Geometry check sheet. Reference: the model listing, model coordinates, mm. Give positions to 0.01 mm unless a question says otherwise; leave off trailing zeros. Order: outer loops, then holes, each group sorted by start corner. A loop starts at its lowest first (then second) coordinate and runs counter-clockwise, first axis right, second up. Notation, with made-up numbers: M 81.25,74.5 L 112.25,74.5 A23 ccw 112.25,102.5 Z; hole C 17.5,32 d1. An arc over 180 degrees is marked long. Answer as CSV lines item,"result". Start each with the question number.
Autodesk Fusion 360 part; units mm, degrees
sketch "ControlPanel" plane through (0, 0, 0) normal (0, 1, 0) x (-1, 0, 0)
  line L0 (0, 0) -> (73, 0)
  line L1 (73, 0) -> (73, 41)
  line L2 (73, 41) -> (0, 41)
  line L3 (0, 41) -> (0, 0)
  line L4 (-11.9813, -5) -> (34.0187, -5)
  line L5 (34.0187, -5) -> (34.0187, -32)
  line L6 (34.0187, -32) -> (-11.9813, -32)
  line L7 (-11.9813, -32) -> (-11.9813, -5)
  line L8 (77.6844, -83.0568) -> (77.6844, -82.5327)
  line L9 (-12.1589, -88.0054) -> (-12.1589, -100.8506)
  line L10 (13.8411, -100.8506) -> (13.8411, -88.0054)
  arc A0 (-12.1589, -100.8506) -> (13.8411, -100.8506) centre (0.8411, -94.428) ccw
  arc A1 (13.8411, -88.0054) -> (-12.1589, -88.0054) centre (0.8411, -94.428) ccw
  line L11 (76.8382, -83.928) -> (70.2808, -83.928)
  line L12 (63.0595, -91.1493) -> (63.0595, -97.7068)
  line L13 (70.2808, -104.928) -> (76.8382, -104.928)
  line L14 (84.0595, -97.7068) -> (84.0595, -91.1493)
  arc A2 (70.2808, -83.928) -> (63.0595, -91.1493) centre (73.5595, -94.428) ccw
  arc A3 (84.0595, -91.1493) -> (76.8382, -83.928) centre (73.5595, -94.428) ccw
  arc A4 (63.0595, -97.7068) -> (70.2808, -104.928) centre (73.5595, -94.428) ccw
  arc A5 (76.8382, -104.928) -> (84.0595, -97.7068) centre (73.5595, -94.428) ccw
  line L15 (39.0187, -5) -> (85.0187, -5)
  line L16 (85.0187, -5) -> (85.0187, -32)
  line L17 (85.0187, -32) -> (39.0187, -32)
  line L18 (39.0187, -32) -> (39.0187, -5)
  line L19 (-11.9813, -37) -> (34.0187, -37)
  line L20 (34.0187, -37) -> (34.0187, -64)
  line L21 (34.0187, -64) -> (-11.9813, -64)
  line L22 (-11.9813, -64) -> (-11.9813, -37)
  line L23 (39.0187, -37) -> (85.0187, -37)
  line L24 (85.0187, -37) -> (85.0187, -64)
  line L25 (85.0187, -64) -> (39.0187, -64)
  line L26 (39.0187, -64) -> (39.0187, -37)
  line L27 (34.0187, -5) -> (39.0187, -5) construction
  circle A6 centre (36.5, -94.428) radius 0.6723 construction
  line L28 (119.0595, -139.428) -> (119.0595, 71) construction
  line L29 (119.0595, 71) -> (-44.1589, 71) construction
  line L30 (-44.1589, 71) -> (-44.1589, -139.428) construction
  line L31 (-44.1589, 71) -> (119.0595, 71)
  line L32 (119.0595, 71) -> (119.0595, -219)
  line L33 (119.0595, -219) -> (-44.1589, -219)
  line L34 (-44.1589, -219) -> (-44.1589, 71)
  circle A7 centre (-14.1589, 61) radius 3
  circle A8 centre (89.0595, 61) radius 3
  circle A9 centre (-34.1589, 31) radius 3
  circle A10 centre (109.0551, 31) radius 3
  circle A11 centre (-34.1589, -19) radius 3
  circle A12 centre (109.0551, -19) radius 3
  circle A13 centre (-34.1589, -69) radius 3
  circle A14 centre (109.0551, -69) radius 3
  circle A15 centre (-34.1589, -119) radius 3
  circle A16 centre (109.0551, -119) radius 3
  circle A17 centre (-34.1589, -169) radius 3
  circle A18 centre (109.0551, -169) radius 3
  circle A19 centre (-14.1589, -209) radius 3
  circle A20 centre (89.0595, -209) radius 3
  point P0 (73.5595, -94.428)
  point P1 (0.8411, -94.428)
  point P2 (73.5595, -94.428)
  point P3 (0.8411, -94.428)
  point P4 (73.5595, -94.428)
  point P5 (-14.1589, -209)
  point P6 (89.0595, -209)
  dimension "d12" = 73
  dimension "d13" = 41
  dimension "d15" = 46
  dimension "d16" = 27
  dimension "d17" = 5
  dimension "d33" = 29
  dimension "d36" = 22
  dimension "d88" = 46
  dimension "d89" = 27
  dimension "d90" = 5
  dimension "d91" = 46
  dimension "d92" = 27
  dimension "d93" = 5
  dimension "d94" = 46
  dimension "d95" = 27
  dimension "d96" = 5
  dimension "d110" = 210.428
  dimension "d111" = 290
  dimension "d113" = 6
  dimension "d114" = 30
  dimension "d115" = 6
  dimension "d116" = 30
  dimension "d123" = 6
  dimension "d124" = 40
  dimension "d127" = 143.214
  dimension "d128" = -200
extrude "Extrude3" add sketch "ControlPanel" along normal blind 3 contours L31 L32 L33 L34 | A19 | A20
extrude "Extrude5" cut sketch "ControlPanel" along normal mid plane 12 contours A19
extrude "Extrude6" cut sketch "ControlPanel" along normal mid plane 12 contours A20
extrude "Extrude1" [suppressed]
equation "m2_w = 73 mm"
equation "m2_h = 41 mm"
equation "m1_w = 46 mm"
equation "m1_h = 27 mm"
equation "mpwr_dia = 12.2 mm"
equation "mpwr_key = 1 mm"
equation "reset_dia = 12.5 mm"
equation "apwr_dia = 29 mm"
equation "apwr_key = 26 mm"
equation "estop_dia = 22 mm"
equation "estop_key = 21 mm"
equation "d12 = m2_w"
equation "d13 = m2_h"
equation "meter_v = 5 mm"
equation "d15 = m1_w"
equation "d16 = m1_h"
equation "d17 = meter_v"
equation "apwr_shell = 37 mm"
equation "botrow_offset = 35 mm"
equation "d33 = apwr_dia"
equation "d36 = estop_dia"
equation "sw_dist = 100 mm"
equation "sw_offs = 25 mm"
equation "text_top_offs = 5 mm"
equation "d88 = m1_w"
equation "d89 = m1_h"
equation "d90 = meter_v"
equation "d91 = m1_w"
equation "d92 = m1_h"
equation "d93 = meter_v"
equation "d94 = m1_w"
equation "d95 = m1_h"
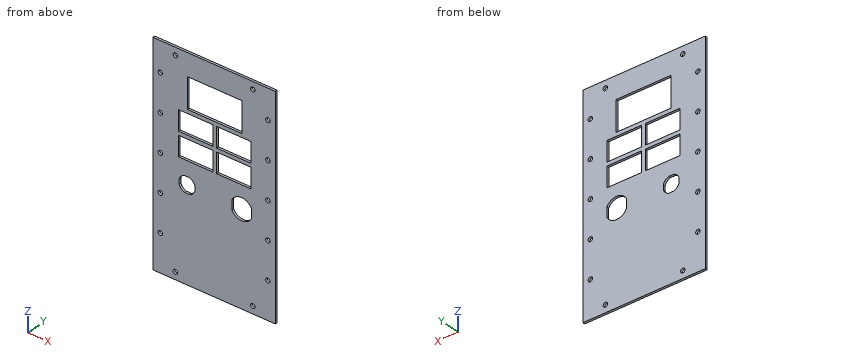
Item 1: Section check A-A on z = 31. Record the boundary of the cut face in (x, y), then the cut area to 3 significant figures.
Item 2: Section check C-C on z = -19. Record the boundary of the cut face in (x, y), then the cut area to 3 significant figures.
Item 3: Section check D-D on z = -169. Record the boundary of the cut face in (x, y), then the cut area to 3 significant figures.
Item 4: Section check B-B on x = -22. Record the boundary of the cut face in (y, z), then the cut area to 3 significant figures.
Item 5: Scan lines: line 1 along Z through (x, y) = (-27, 1.15); line 2 along Z through (x, y) = (34.5, 2); line 3 along X through (y, z) = (1.6, -57.5). Record each from-to range of solid material in increasing order.
Item 6: Depth check by flat-ended pin: pin 1 Ø3.5 at (x, z) = (-109.06, -19) entering from -Y. Enter the tip coordinate at first touch or a pass-through.
Numbers:
1,outline,"M -119.06,0 L -112.06,0 L -112.06,3 L -119.06,3 Z; M -106.06,0 L -73,0 L -73,3 L -106.06,3 Z; M 0,0 L 31.16,0 L 31.16,3 L 0,3 Z; M 37.16,0 L 44.16,0 L 44.16,3 L 37.16,3 Z"
1,area,"235 mm2"
2,outline,"M -119.06,0 L -112.06,0 L -112.06,3 L -119.06,3 Z; M -106.06,0 L -85.02,0 L -85.02,3 L -106.06,3 Z; M -39.02,0 L -34.02,0 L -34.02,3 L -39.02,3 Z; M 11.98,0 L 31.16,0 L 31.16,3 L 11.98,3 Z; M 37.16,0 L 44.16,0 L 44.16,3 L 37.16,3 Z"
2,area,"178 mm2"
3,outline,"M -119.06,0 L -112.06,0 L -112.06,3 L -119.06,3 Z; M -106.06,0 L 31.16,0 L 31.16,3 L -106.06,3 Z; M 37.16,0 L 44.16,0 L 44.16,3 L 37.16,3 Z"
3,area,"454 mm2"
4,outline,"M 0,-219 L 3,-219 L 3,-64 L 0,-64 Z; M 0,-37 L 3,-37 L 3,-32 L 0,-32 Z; M 0,-5 L 3,-5 L 3,0 L 0,0 Z; M 0,41 L 3,41 L 3,71 L 0,71 Z"
4,area,"585 mm2"
5,line 1,"-219 to -64, -37 to -32, -5 to 0, 41 to 71"
5,line 2,"-219 to -171.98, -166.02 to -121.98, -116.02 to -71.98, -66.02 to -21.98, -16.02 to 28.02, 33.98 to 71"
5,line 3,"-119.06 to -85.02, -39.02 to -34.02, 11.98 to 44.16"
6,pin 1,"through"
